Build history of the part. All positions in model axes, mm. A direction names the side the tool comes from. Give positions to 0.01 mm unless a question says otherwise; leave off trailing zeros. Write each loop counter-clockwise with the first axis right and the second up, starting at its lowest first coordinate (ties: lowest second). Pieces come first, ordered by that corner, then holes. Notation, with made-up numbers: M 88,2 L 115,2 A27 ccw 115,22 Z; hole C 25,-6 d7. An arc over 180 degrees is marked long. One line per item, written item: value. Start each with the question number.
Autodesk Inventor part; units mm, degrees
ref_plane "YZ Plane" through (0, 0, 0) normal (1, 0, 0) x (0, 1, 0)
ref_plane "XZ Plane" through (0, 0, 0) normal (0, 1, 0) x (-1, 0, 0)
ref_plane "XY Plane" through (0, 0, 0) normal (0, 0, 1) x (1, 0, 0)
sketch "Sketch1" plane through (0, 0, 0) normal (0, 0, 1) x (1, 0, 0)
  line L0 (0, 0) -> (-40, 0)
  line L1 (-40, 0) -> (-40, 20)
  line L2 (-40, 20) -> (0, 20)
  line L3 (0, 20) -> (0, 0)
  dimension "d0" = 40
  dimension "d1" = 20
extrude "Extrusion1" add sketch "Sketch1" along normal blind 20
sketch "Sketch2" plane through (-40, 20, 0) normal (0, 1, 0) x (1, 0, 0)
  line L0 (0, -20) -> (40, -20)
  line L1 (40, -20) -> (40, -16)
  line L2 (40, 0) -> (40, -20)
  line L3 (28, -20) -> (28, -16)
  line L4 (28, -16) -> (40, -16)
  dimension "d4" = 4
  dimension "d5" = 12
extrude "Extrusion2" cut sketch "Sketch2" against normal through all
sketch "Sketch3" plane through (0, 0, 0) normal (1, 0, 0) x (0, 0, -1)
  line L0 (-16, 20) -> (-16, 0)
  line L1 (-16, 12) -> (0, 12)
  line L2 (0, 20) -> (0, 0)
  line L3 (0, 8) -> (-16, 8)
  dimension "d8" = 8
  dimension "d9" = 8
extrude "Extrusion3" cut sketch "Sketch3" against normal blind 12
sketch "Sketch4" plane through (-40, 20, 0) normal (0, 1, 0) x (1, 0, 0)
  circle A0 centre (32, -8) radius 2.25
  line L0 (28, -16) -> (40, -16)
  line L1 (40, 0) -> (40, -16)
  dimension "d12" = 4.5
  dimension "d13" = 8
  dimension "d14" = 8
extrude "Extrusion4" cut sketch "Sketch4" against normal through all
sketch "Sketch5" plane through (-40, 0, 0) normal (0, -1, 0) x (1, 0, 0)
  line L0 (40, 0) -> (40, 16)
  line L1 (0, 0) -> (0, 20)
  line L2 (40, 0) -> (32, 0)
  line L3 (32, 12.1569) -> (35.6, 10.0785)
  line L4 (35.6, 10.0785) -> (35.6, 5.9215)
  line L5 (35.6, 5.9215) -> (32, 3.8431)
  line L6 (32, 3.8431) -> (28.4, 5.9215)
  line L7 (28.4, 5.9215) -> (28.4, 10.0785)
  line L8 (28.4, 10.0785) -> (32, 12.1569)
  line L9 (40, 16) -> (28, 16)
  dimension "d28" = 7.2
  dimension "d29" = 4.4
  dimension "d30" = 3.8431
  dimension "d31" = 3.8431
  dimension "d32" = 2.0785
  dimension "d33" = 4.1569
  dimension "d34" = 2.0785
extrude "Extrusion5" cut sketch "Sketch5" against normal blind 4
sketch "Sketch6" plane through (-40, 20, 0) normal (0, 1, 0) x (1, 0, 0)
  circle A0 centre (32, -8) radius 4
  line L0 (28, -16) -> (40, -16)
  line L1 (40, 0) -> (40, -16)
  dimension "d37" = 8
  dimension "d38" = 8
  dimension "d39" = 8
extrude "Extrusion6" cut sketch "Sketch6" against normal blind 4
properties part number "connectiontest1"
1) Band-saw the part on A-A (z = 8). List the corners of the cut face in (x, y).
2) Tool access for faces 4 (the face through (-6, 16, 16)), 5 (the face through (-4.4, 2, 8)), 6 (the face through (-11.2, 18, 10.4)), 7 (the face through (-5, 12, 8)), 8 (the face through (-12, 11, 14)): list every direction of +Z, -Z, +X, -X, +Y, -Y with a clear straight run to the whole face (end or side of a thin tool).
3) Band-saw the part on D-D (y = 9.75). List the corners of the cut face in (x, z).
4) Drop flat-ended pins along their axis: P1, Ø2.5, axis at x = -8, z = 8, coming from the +Y side; P2, Ø3, axis at x = -4.5, y = 9, coming from the +Z side; P3, Ø12, axis at y = 6.5, z = 7, coming from the +X side; P4, Ø1, axis at x = -6, z = 10, coming from the +Y side. Give the stop position or say it passes through.
5) Band-saw the part on B-B (y = 14). List the corners of the cut face in (x, z), then the cut area to 3 significant figures.
6) Mould opens along X. For faces 1 (the face through (-26, 10, 20)), 2 (the face through (-9.66, 14.03, 6.48)), 3 (the face through (0, 4, 8)) say: released by +X, released by -X, zero draft, split by the parting line, or undercut.
7) Probe line 1 along X through (y, z) = (1.25, 8.75); line 2 along Y through (x, z) = (-9, 14.5); line 3 along Z through (x, y) = (-8, 16.9). List the from-to ranges inside material, lowest first. Write a range as from..to.
8) Band-saw the part on C-C (z = 1.5). List the corners of the cut face in (x, y), then the cut area to 3 significant figures.
Model answer:
1. outline: M -40,0 L -11.6,0 L -11.6,4 L -10.25,4 L -10.25,8 L -12,8 L -12,12 L -10.25,12 L -10.25,16 L -12,16 L -12,20 L -40,20 Z; M -5.75,4 L -4.4,4 L -4.4,0 L 0,0 L 0,8 L -5.75,8 Z; M -5.75,12 L 0,12 L 0,20 L -4,20 L -4,16 L -5.75,16 Z
2. face 4: +Z, +X, +Y, -Y
2. face 5: -Y
2. face 6: +Y
2. face 7: +Z, -Z, +X
2. face 8: +Z, +X
3. outline: M -40,0 L -12,0 L -12,20 L -40,20 Z
4. P1: passes through
4. P2: stops at z = 16
4. P3: stops at x = 0
4. P4: stops at y = 16
5. outline: M -40,0 L 0,0 L 0,16 L -12,16 L -12,20 L -40,20 Z; hole C -8,8 d4.5
5. area: 736 mm²
6. face 1: zero draft
6. face 2: undercut
6. face 3: released by +X
7. line 1: x = -40..-11.6, -4.4..0
7. line 2: y = 0..8, 12..20
7. line 3: z = 0..4, 12..16
8. outline: M -40,0 L 0,0 L 0,8 L -12,8 L -12,12 L 0,12 L 0,20 L -40,20 Z
8. area: 752 mm²
